```python
from build123d import *

# Parameters (mm, degrees)
SKETCH1_W                   = 135
SKETCH1_H                   = 110
BOSS_EXTRUDE1_DEPTH         = 100
BOSS_EXTRUDE2_DEPTH         = 29.999999629
BOSS_EXTRUDE3_START         = 30.000000371
BOSS_EXTRUDE3_DEPTH         = 30.000000371
SKETCH4_W                   = 135
SKETCH4_H                   = 100
BOSS_EXTRUDE4_DEPTH         = 30
BOSS_EXTRUDE5_DEPTH         = 55
SKETCH6_W                   = 20
SKETCH6_H                   = 160
BOSS_EXTRUDE6_DEPTH         = 5
SKETCH7_W                   = 20
SKETCH7_H                   = 160
BOSS_EXTRUDE7_DEPTH         = 5
CUT_EXTRUDE1_START          = -29.999999629
CUT_EXTRUDE1_DEPTH          = 29.999999629
CUT_EXTRUDE2_DEPTH          = 30.000000371
SKETCH10_W                  = 35
SKETCH10_H                  = 40
CUT_EXTRUDE3_DEPTH          = 30
HOLE1_D                     = 80
HOLE1_DEPTH                 = 135
HOLE2_REACH                 = 255.032
HOLE2_BORE_R                = 30
F_3_4_CLEARANCE_HOLE1_D     = 20
F_3_4_CLEARANCE_HOLE1_DEPTH = 24.602326997
F_3_4_CLEARANCE_HOLE2_D     = 20
FILLET1_R                   = 5
FILLET2_R                   = 10


with BuildPart() as part:
    # Sketch1 → Boss-Extrude1 (new body)
    with BuildSketch(Plane(origin=(0, 50.000000371, 0), x_dir=(1, 0, 0), z_dir=(0, 1, 0))):
        with Locations((-27.5, -55)):
            Rectangle(SKETCH1_W, SKETCH1_H)
    extrude(amount=-BOSS_EXTRUDE1_DEPTH)

    # Sketch2 → Boss-Extrude2 (add)
    with BuildSketch(Plane(origin=(0, 50.000000371, 0), x_dir=(-1, 0, 0), z_dir=(0, 1, 0))):
        with BuildLine():
            Line((-40, 0), (-40, 110))
            ThreePointArc((-40, 110), (20.288540009, 65.716947722), (95, 61.989412153))
            Line((95, 61.989412153), (95, 0))
            Line((95, 0), (-40, 0))
        make_face()
    extrude(amount=BOSS_EXTRUDE2_DEPTH)

    # Sketch3 → Boss-Extrude3 (add)
    with BuildSketch(Plane.XZ.offset(49.999999629).offset(BOSS_EXTRUDE3_START)):
        with BuildLine():
            Line((40, 0), (-95, 0))
            Line((-95, 0), (-95, 61.989412153))
            ThreePointArc((-95, 61.989412153), (-20.288540009, 65.716947722), (40, 110))
            Line((40, 110), (40, 0))
        make_face()
    extrude(amount=-BOSS_EXTRUDE3_DEPTH)

    # Sketch4 → Boss-Extrude4 (add)
    with BuildSketch(Plane.XY.offset(110)):
        with Locations((-27.5, 3.71e-07)):
            Rectangle(SKETCH4_W, SKETCH4_H)
    extrude(amount=BOSS_EXTRUDE4_DEPTH)

    # Sketch5 → Boss-Extrude5 (add)
    with BuildSketch(Plane(origin=(40, 0, 0), x_dir=(0, 0, -1), z_dir=(1, 0, 0))):
        Polygon((-140, 50.000000371), (-20, 50.000000371), (-20, 80), (0, 80), (0, -80), (-20, -80), (-20, -49.999999629), (-140, -49.999999629), align=None)
    extrude(amount=BOSS_EXTRUDE5_DEPTH)

    # Sketch6 → Boss-Extrude6 (add)
    with BuildSketch(Plane.ZY.offset(95)):
        with Locations((10, 0)):
            Rectangle(SKETCH6_W, SKETCH6_H)
    extrude(amount=BOSS_EXTRUDE6_DEPTH)

    # Sketch7 → Boss-Extrude7 (add)
    with BuildSketch(Plane(origin=(95, 0, 0), x_dir=(0, 0, -1), z_dir=(1, 0, 0))):
        with Locations((-10, 0)):
            Rectangle(SKETCH7_W, SKETCH7_H)
    extrude(amount=BOSS_EXTRUDE7_DEPTH)

    # Sketch8 → Cut-Extrude1 (cut)
    with BuildSketch(Plane(origin=(0, 80, 0), x_dir=(-1, 0, 0), z_dir=(0, 1, 0)).offset(CUT_EXTRUDE1_START)):
        with BuildLine():
            Line((47.874205856, 59.186990419), (47.874205856, 30))
            Line((47.874205856, 30), (95, 30))
            Line((95, 30), (95, 61.989412153))
            ThreePointArc((95, 61.989412153), (71.565380287, 58.431076847), (47.874205856, 59.186990419))
        make_face()
    extrude(amount=CUT_EXTRUDE1_DEPTH, mode=Mode.SUBTRACT)

    # Sketch9 → Cut-Extrude2 (cut)
    with BuildSketch(Plane.XZ.offset(80)):
        with BuildLine():
            Line((-47.874205856, 30), (-47.874205856, 59.186990419))
            ThreePointArc((-47.874205856, 59.186990419), (-71.565380287, 58.431076847), (-95, 61.989412153))
            Line((-95, 61.989412153), (-95, 30))
            Line((-95, 30), (-47.874205856, 30))
        make_face()
    extrude(amount=-CUT_EXTRUDE2_DEPTH, mode=Mode.SUBTRACT)

    # Sketch10 → Cut-Extrude3 (cut)
    with BuildSketch(Plane(origin=(95, 0, 0), x_dir=(0, 0, -1), z_dir=(1, 0, 0))):
        with Locations((-42.102326997, -1.102144565)):
            Rectangle(SKETCH10_W, SKETCH10_H)
    extrude(amount=-CUT_EXTRUDE3_DEPTH, mode=Mode.SUBTRACT)

    # Hole1
    with Locations(Plane(origin=(0, 0, 0), x_dir=(-1, 0, 0), z_dir=(0, 0, -1))):
        with Locations((0, 0)):
            Hole(HOLE1_D / 2, depth=HOLE1_DEPTH)

    # Hole2 bore → Hole2 (cut, up to next)
    with BuildSketch(Plane(origin=(95, 0, 0), x_dir=(0, 0, -1), z_dir=(1, 0, 0)), mode=Mode.PRIVATE) as hole2_sk1:
        with Locations((-99.999999554, 3.71e-07)):
            Circle(HOLE2_BORE_R)
    hole2_tool1 = extrude(hole2_sk1.sketch, amount=-HOLE2_REACH, mode=Mode.PRIVATE) & part.part
    add(hole2_tool1.solids().sort_by_distance((95, 0, 100))[0], mode=Mode.SUBTRACT)

    # 3/4 Clearance Hole1
    with Locations(Plane.XY.offset(24.602326997)):
        with Locations((83.46, 0.37)):
            Hole(F_3_4_CLEARANCE_HOLE1_D / 2, depth=F_3_4_CLEARANCE_HOLE1_DEPTH)

    # 3/4 Clearance Hole2 (through all)
    with Locations(Plane.XY.offset(30)):
        with Locations((-77.895356155, -62.316284924), (-77.895356155, 62.316284924)):
            Hole(F_3_4_CLEARANCE_HOLE2_D / 2)

    # Fillet1
    fillet1_edges = [part.edges().sort_by_distance(p)[0] for p in [
        (-100, -80, 10),
        (-100, 80, 10),
        (100, -80, 10),
        (100, 80, 10),
    ]]
    fillet(fillet1_edges, radius=FILLET1_R)

    # Fillet2
    fillet2_edges = [part.edges().sort_by_distance(p)[0] for p in [
        (1.227361836, 80, 75.662254106),
        (-47.874205856, 65.000000185, 59.186990419),
        (-47.874205856, 80, 44.593495209),
        (-95, -80, 25),
        (-47.874205856, -64.999999815, 59.186990419),
        (-47.874205856, -80, 44.593495209),
        (-95, 50.000000371, 85),
        (95, -21.102144565, 42.102326997),
        (95, 18.897855435, 42.102326997),
        (95, -1.102144565, 59.602326997),
        (40, 65.000000185, 110),
        (40, 80, 65),
        (-95, -49.999999629, 85),
        (40, -64.999999815, 110),
        (1.227361836, -80, 75.662254106),
        (0, 50.000000371, 140),
        (-95, 3.71e-07, 140),
        (0, -49.999999629, 140),
        (40, -80, 65),
        (-95, 80, 25),
    ]]
    fillet(fillet2_edges, radius=FILLET2_R)


solid = part.part
```
Check sheet for the modelled part. Datum: model origin and axes. Units: mm. A direction names the side the tool comes from. Coordinates: 2 decimals unless noted, no trailing zeros. Order: outer loops, then holes, each group sorted by start corner. A loop starts at its lowest first (then second) coordinate and runs counter-clockwise, first axis right, second up. Notation, with made-up numbers: M -5,51 L 10,51 A19 ccw 10,58 Z; hole C 15.25,3 d3. An arc over 180 degrees is marked long. Write each question's results on one line, items separated by ' | '. Start each with the question number.
1. Cross-section at D-D on z = 9.5. Record the cut outline in (x, y), and give its area (3 significant figures).
2. Access from +Z, -Z, +X, -X, +Y, -Y to the whole of each face (thin tool, end or side, straight path). Record for faces 4 (the face through (34.207, 60.14, 93.387)), 5 (the face through (-95, -1, 74)), 6 (the face through (36.99, -77.15, 51.71)), 7 (the face through (-6.51, -60.14, 71.53)).
3. Material ranges on probe 1 along Z at (x, y) = (62, 1); probe 2 along Y at (x, z) = (-48.5, 56); probe 3 along Y at (x, z) = (83.46, 13), recorded low to high.
4. Cross-section at B-B on y = 26. Record the cut outline in (x, z).
5. Go/stop test with flat-tipped pins: P1, Ø5, axis at y = 8.5, z = 89, coming from the +X side; P2, Ø16, axis at y = 55.5, z = 36, coming from the -X side; P3, Ø22, axis at y = -58.5, z = 65, coming from the +X side; P4, Ø16, axis at x = 74.5, y = -10, coming from the -Z side. Record where each tip stops, or that it passes through.
6. Cross-section at C-C on z = 27.5. Record the cut outline in (x, y), and give its area (3 significant figures).
7. Cross-section at A-A on z = 100. Record the cut outline in (x, y), and give its area (3 significant figures).
8. Mould release check, pull along Y, two halves, no side actions. Record for faces 1 (the face through (-44.867, 77.148, 40.172)), 2 (the face through (-98, -79, 10)), 3 (the face through (-39.96, 1.76, 68.44)): +Y half, -Y half, draft (parallel to the pull), parting line (faces both ways), or undercut.
Checks:
1) outline: M -100,-75 A5 ccw -95,-80 L 95,-80 A5 ccw 100,-75 L 100,75 A5 ccw 95,80 L -95,80 A5 ccw -100,75 Z; hole C -77.9,-62.32 d20; hole C -77.9,62.32 d20; hole C 0,0 d80; hole C 83.46,0.37 d20 | area: 26,000 mm²
2) face 4: +Z, +Y | face 5: +Z, -X, +Y, -Y | face 6: +Z, +X, -Y | face 7: +Z, -X, -Y
3) probe 1: z = 0 to 70.02, 129.98 to 140 | probe 2: y = -50 to 50 | probe 3: y = -80 to -9.63, 10.37 to 80
4) outline: M -100,0 L -30.4,0 L -30.4,135 L 30.4,135 L 30.4,114.97 L 95,114.97 L 95,140 L -85,140 A10 ccw -95,130 L -95,20 L -100,20 Z; M 30.4,0 L 100,0 L 100,20 L 95,20 L 95,24.6 L 94.57,24.6 L 94.57,66.7 A10 ccw 95,69.6 L 95,85.03 L 30.4,85.03 Z
5) P1: stops at x = -38.46 | P2: stops at x = -95 | P3: stops at x = 95 | P4: stops at z = 0
6) outline: M -95,-70 A10 ccw -85,-80 L 30,-80 A10 ccw 40,-70 L 40,-50 L 95,-50 L 95,-31.1 A10 ccw 85,-21.1 L 65,-21.1 L 65,18.9 L 85,18.9 A10 ccw 95,28.9 L 95,50 L 40,50 L 40,70 A10 ccw 30,80 L -85,80 A10 ccw -95,70 Z; hole C -77.9,-62.32 d20; hole C -77.9,62.32 d20; hole C 0,0 d80 | area: 20,100 mm²
7) outline: M -95,-40 A10 ccw -85,-50 L 95,-50 L 95,-30 L 26.46,-30 A40 cw long 26.46,30 L 95,30 L 95,50 L -85,50 A10 ccw -95,40 Z | area: 10,400 mm²
8) face 1: +Y half | face 2: -Y half | face 3: undercut
